Print and shaded views of the part. All mm, measured from the part's lowest x, y and z. A direction names the side the tool comes from. Coordinates: 2 decimals unless noted, no trailing zeros. Order: outer loops, then holes, each group sorted by start corner. A loop starts at its lowest first (then second) coordinate and runs counter-clockwise, first axis right, second up. Notation, with made-up numbers: M 31,-35.5 L 35,-35.5 A25 cw 35,-15.5 Z; hole C 30,-2.5 d9. An arc over 180 degrees is marked long. One line per item, written item: value.
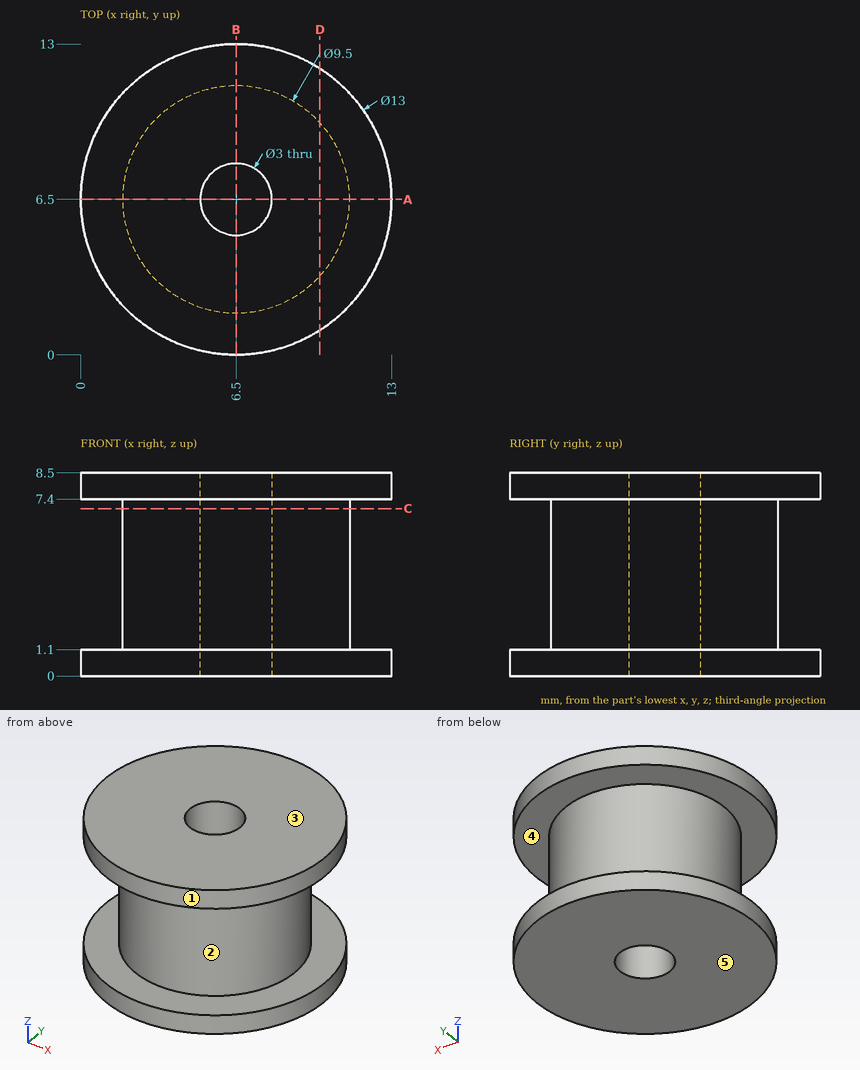
Q1. Mould opens along Z. For the marked faces 1, 2 and 3 say: released by +Z, released by -Z, zero draft, split by the parting line, or undercut.
Recorded:
face 1: zero draft
face 2: undercut
face 3: released by +Z
Q2. Which spindle directions (+Z, -Z, +X, -X, +Y, -Y) get a long thin tool onto all of the face, cutting with end or side? Do the marked faces 4 and 5. Say none if no direction does.
Recorded:
face 4: none
face 5: -Z, +X, -X, +Y, -Y
Q3. Slice it at D-D (x = 10). List the corners of the cut face in (y, z).
Recorded:
outline: M 1.02,0 L 11.98,0 L 11.98,1.1 L 9.71,1.1 L 9.71,7.4 L 11.98,7.4 L 11.98,8.5 L 1.02,8.5 L 1.02,7.4 L 3.29,7.4 L 3.29,1.1 L 1.02,1.1 Z
Q4. Pin check, flat tips, straight feed: pin 1 Ø1.5 at (x, z) = (11, 5.5) entering from +Y; pin 2 Ø4 at (x, z) = (3, 6) entering from -Y; pin 3 Ø1 at (x, z) = (4.5, 6.5) entering from +Y. Stop position of each tip, or through.
Recorded:
pin 1: stops at y = 9.42
pin 2: stops at y = 0.34
pin 3: stops at y = 11.01
Q5. Slice it at A-A (y = 6.5). List the corners of the cut face in (x, z).
Recorded:
outline: M 0,0 L 5,0 L 5,8.5 L 0,8.5 L 0,7.4 L 1.75,7.4 L 1.75,1.1 L 0,1.1 Z; M 8,0 L 13,0 L 13,1.1 L 11.25,1.1 L 11.25,7.4 L 13,7.4 L 13,8.5 L 8,8.5 Z
Q6. Slice it at C-C (z = 7). List the corners of the cut face in (x, y).
Recorded:
outline: C 6.5,6.5 d9.5; hole C 6.5,6.5 d3
Q7. Drill centre lines: line 1 along Z through (x, y) = (9.75, 12); line 2 along Y through (x, z) = (6.5, 6.75); line 3 along Y through (x, z) = (7.75, 7.5). Where is each one in solid material? Low to high.
Recorded:
line 1: z = 0 to 1.1, 7.4 to 8.5
line 2: y = 1.75 to 5, 8 to 11.25
line 3: y = 0.12 to 5.67, 7.33 to 12.88
